```python
from build123d import *

# Parameters (mm, degrees)
F0_W     = 100
F0_H     = 100
F0_R     = 31
F1_DEPTH = 38.44
F2_R     = 6
F3_DEPTH = 19.5871874485


with BuildPart() as f1:
    # F0 (on Front) → F1 (new body)
    with BuildSketch(Plane.XZ):
        Rectangle(F0_W, F0_H)
        Circle(F0_R, mode=Mode.SUBTRACT)
    extrude(amount=F1_DEPTH)

    # F2 (on face) → F3 (cut, through all)
    with BuildSketch(Plane(origin=(0, 0, -50), x_dir=(1, 0, 0), z_dir=(0, 0, -1))):
        with Locations((0, 19.22)):
            Circle(F2_R)
    extrude(amount=-F3_DEPTH, mode=Mode.SUBTRACT)


solid = f1.part
```
Can you work these out from the model? Positions are in its coordinate system, mm. Give positions to 0.01 mm unless a question says otherwise; leave off trailing zeros. Loops run counter-clockwise (first coordinate to the right, second up) from the corner with the lowest first, then second, coordinate; pieces in that order, holes last. Notation, with made-up numbers: M 31,15.5 L 65,15.5 A22 ccw 65,38.5 Z; hole C 74,-8 d4. An arc over 180 degrees is marked long. Answer in a Markdown table with one row per item.
1. Suppose I cut it at A-A on x = 0. Write out the boundary of the cut face in (y, z).
Taken from the geometry:
| item | result |
|---|---|
| outline | M -38.44,-50 L -25.22,-50 L -25.22,-31 L -38.44,-31 Z; M -38.44,31 L 0,31 L 0,50 L -38.44,50 Z; M -13.22,-50 L 0,-50 L 0,-31 L -13.22,-31 Z |
2. Suppose I cut it at B-B on z = 0. Write out the boundary of the cut face in (x, y), plus the area to 3 significant figures.
Taken from the geometry:
| item | result |
|---|---|
| outline | M -50,-38.44 L -31,-38.44 L -31,0 L -50,0 Z; M 31,-38.44 L 50,-38.44 L 50,0 L 31,0 Z |
| area | 1,460 mm² |
3. Suppose I cut it at C-C on y = -19.22. Write out the boundary of the cut face in (x, z).
Taken from the geometry:
| item | result |
|---|---|
| outline | M -50,-50 L -6,-50 L -6,-30.41 A31 cw long 6,-30.41 L 6,-50 L 50,-50 L 50,50 L -50,50 Z |
4. For pin 1 Ø10 at (x, z) = (24.5, 36) entering from +Y; pin 2 Ø5 at (x, z) = (20, -19) entering from -Y, each with a flat end and sliding along its axis, tell me the tip position at first contact or that it passes through.
Taken from the geometry:
| item | result |
|---|---|
| pin 1 | stops at y = 0 |
| pin 2 | passes through |
5. Suppose I cut it at D-D on x = -25.5. Write out the boundary of the cut face in (y, z).
Taken from the geometry:
| item | result |
|---|---|
| outline | M -38.44,-50 L 0,-50 L 0,-17.63 L -38.44,-17.63 Z; M -38.44,17.63 L 0,17.63 L 0,50 L -38.44,50 Z |
6. If I drill on line 1 along Z through (x, y) = (1, -6.5); line 2 along Y through (x, z) = (0, -38.75); line 3 along X through (y, z) = (-19.22, -39.5), over which ranges is the centre line in solid material (lowest first)?
Taken from the geometry:
| item | result |
|---|---|
| line 1 | z = -50 to -30.98, 30.98 to 50 |
| line 2 | y = -38.44 to -25.22, -13.22 to 0 |
| line 3 | x = -50 to -6, 6 to 50 |
7. Thinking about a two-plate mould opening in Y: for faces 1 (the flat face through (-1, -19, 50)), 2 (the cylindrical face through (-0.78, -25.17, -40.34)), 3 (the flat face through (-23, 0, 23)), which applies, released by +Y, released by -Y, zero draft, split by the parting line, or undercut?
Taken from the geometry:
| item | result |
|---|---|
| face 1 | zero draft |
| face 2 | undercut |
| face 3 | released by +Y |
